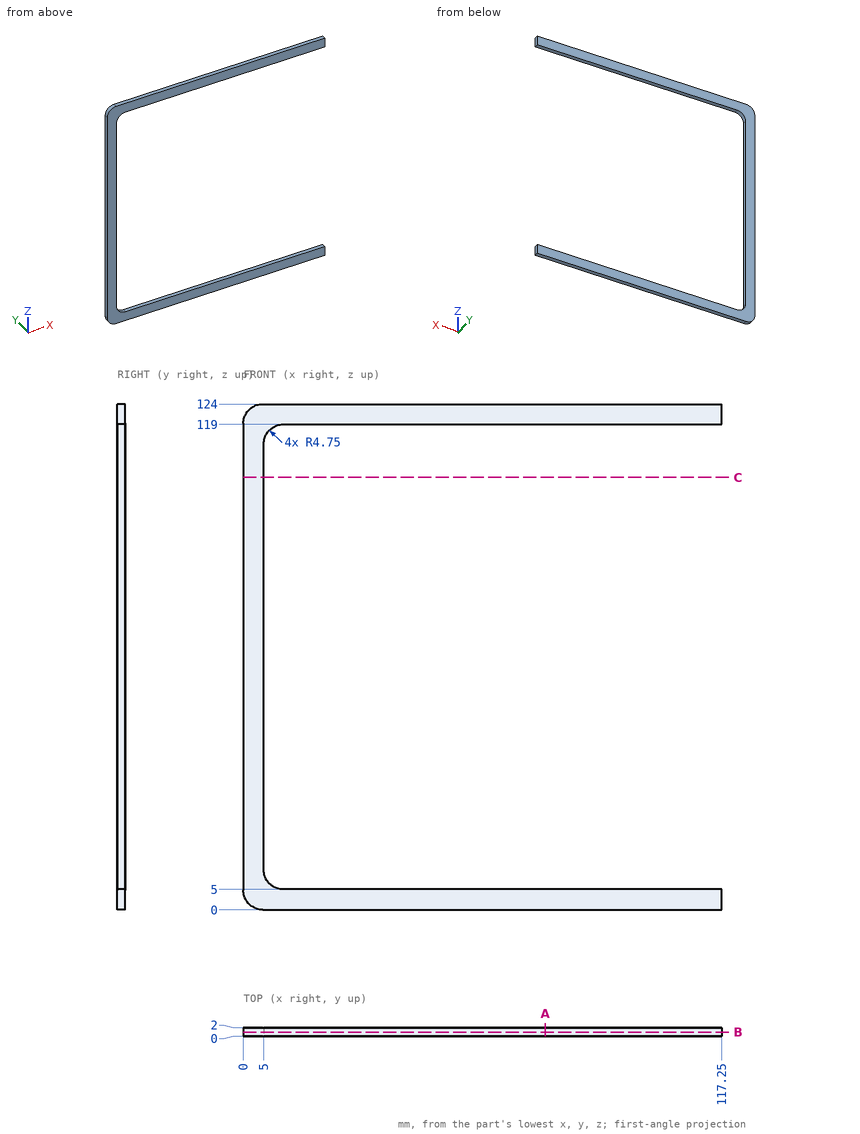
Design review of the part shown in the three views and the two pictorial views. Dimensions are in mm from the part's minimum x, y and z. Coordinates: 2 decimals unless noted, no trailing zeros. Write each loop counter-clockwise with the first axis right and the second up, starting at its lowest first coordinate (ties: lowest second). Pieces come first, ordered by that corner, then holes. Notation, with made-up numbers: (73.5, 75) - (98.5, 75) arc R12 cw to (98.5, 89) - close; hole circle Ø6 at (61.25, 28). An arc over 180 degrees is marked (long way). Write item = value, one per line.
(1) Consider section A-A, the plane x = 74. Give the boundary of the cut face in (y, z).
Result sheet:
outline = (0, 0) - (2, 0) - (2, 5) - (0, 5) - close; (0, 119) - (2, 119) - (2, 124) - (0, 124) - close
(2) For line 1 (Z direction, x = 14, y = 1.8); line 2 (X direction, y = 1.05, z = 61); line 3 (X direction, y = 0.75, z = 117), list the stretches that pass through material, from the lowest coordinate up. Write a range as [from, to].
Result sheet:
line_1 = [0, 5], [119, 124]
line_2 = [0, 5]
line_3 = [0, 5.88]
(3) Consider section C-C, the plane z = 106. Give the boundary of the cut face in (x, y), then the cut area to 3 significant figures.
Result sheet:
outline = (0, 0) - (5, 0) - (5, 2) - (0, 2) - close
area = 10.0 mm^2
(4) For P1, Ø1, axis at y = 0.5, z = 73, coming from the +X side, flat-tipped, find the tip position at first contact; note if it passes through.
Result sheet:
P1 = 5
(5) Consider section B-B, the plane y = 0.95. Give the boundary of the cut face in (x, z), then the cut area to 3 significant figures.
Result sheet:
outline = (0, 4.75) arc R4.75 ccw to (4.75, 0) - (117.25, 0) - (117.25, 5) - (9.75, 5) arc R4.75 cw to (5, 9.75) - (5, 114.25) arc R4.75 cw to (9.75, 119) - (117.25, 119) - (117.25, 124) - (4.75, 124) arc R4.75 ccw to (0, 119.25) - close
area = 1,740 mm^2
